```python
from build123d import *

# Parameters (mm, degrees)
SKETCH1_W                 = 25
SKETCH1_H                 = 10
CUT_EXTRUDE1_DEPTH        = 37.742346142
CUT_EXTRUDE1_DEPTH_BACK   = 37.742346142
SKETCH2_R                 = 105
F_3_0MM_DOWEL_HOLE1_D     = 3
F_3_0MM_DOWEL_HOLE1_DEPTH = 6


with BuildPart() as part:
    # Sketch1 → Revolve1 (revolve)
    with BuildSketch(Plane.XY, mode=Mode.PRIVATE) as revolve1_sk:
        with Locations((12.5, 5)):
            Rectangle(SKETCH1_W, SKETCH1_H)
    revolve(revolve1_sk.sketch.rotate(Axis((0, 0, 0), (0, 1, 0)), 90), axis=Axis((0, 0, 0), (0, 1, 0)))

    # Sketch2 → Cut-Extrude1 (cut, two sides: drawn at the far end of the back side and taken through both)
    with BuildSketch(Plane.XY.offset(-CUT_EXTRUDE1_DEPTH_BACK)):
        with Locations((0, 113)):
            Circle(SKETCH2_R)
    extrude(amount=CUT_EXTRUDE1_DEPTH + CUT_EXTRUDE1_DEPTH_BACK, mode=Mode.SUBTRACT)

    # Ø3.0mm Dowel Hole1
    with Locations(Plane(origin=(0, 0, 0), x_dir=(-1, 0, 0), z_dir=(0, -1, 0))):
        with Locations((17, 0)):
            Hole(F_3_0MM_DOWEL_HOLE1_D / 2, depth=F_3_0MM_DOWEL_HOLE1_DEPTH)


solid = part.part
```
The listing builds one solid part. Answer for the finished solid, in the listing's coordinates (mm). A direction names the side the tool comes from. Coordinates: 2 decimals unless noted, no trailing zeros. Loops run counter-clockwise (first coordinate to the right, second up) from the corner with the lowest first, then second, coordinate; pieces in that order, holes last. Notation, with made-up numbers: (-21, 19) -> (-16, 19) arc R21 ccw to (-16, 52) -> close; hole circle Ø5 at (18, 89.5). An arc over 180 degrees is marked (long way). Return JSON: item names as keys, results as strings. Group by question number.
(1) A cutting plane is placed at C-C on y = 6.75. Write down the section's boundary in (x, z).
(2) Given pin 1 Ø2 at (x, z) = (-16, -11) entering from +Y; pin 2 Ø2.5 at (x, z) = (-17, 0) entering from -Y; pin 3 Ø4 at (y, z) = (5, -7.5) entering from -X; pin 4 Ø4 at (x, z) = (19.5, -14) entering from +Y, each flat-ended and moving along its own axis, determine where each tip first touches the part or whether it passes through.
(3) Which of the six approach directions +Z, -Z, +X, -X, +Y, -Y give full straight-line access (tool end or side, diameter ignored) to faces 4 (the flat face through (-22, 10, 0)), 5 (the cylindrical face through (-18.5, 3.04, -0.07))?
(4) Determine the mould class of faces 1 (the cylindrical face through (9.58, 5.07, -23.09)), 2 (the flat face through (22, 10, 0)), 3 (the cylindrical face through (0, 8, 0)) for opening direction X: released by +X, released by -X, zero draft, split by the parting line, or undercut.
(5) A cutting plane is placed at B-B on y = 1.5. Write down the section's boundary in (x, z), and give its area (3 significant figures).
(6) A cutting plane is placed at A-A on z = 0. Write down the section's boundary in (x, y), and give its area (3 significant figures).
(7) Find the intervals of material crossed by probe 1 along Z at (x, y) = (-17, 4.65); probe 2 along X at (y, z) = (7, 15); probe 3 along Y at (x, z) = (-3, 23), in increasing order. Write a range as from..to.
(8) A cutting plane is placed at D-D on x = -17. Write down the section's boundary in (y, z), and give its area (3 significant figures).
The answers:
{
 "1": {"outline": "circle Ø50 at (0, 0)"},
 "2": {"pin 1": "stops at y = 9.39", "pin 2": "stops at y = 6", "pin 3": "stops at x = -24.39", "pin 4": "stops at y = 10"},
 "3": {"face 4": "+Z, -Z, +X, -X, +Y", "face 5": "-Y"},
 "4": {"face 1": "split by the parting line", "face 2": "zero draft", "face 3": "undercut"},
 "5": {"outline": "circle Ø50 at (0, 0); hole circle Ø3 at (-17, 0)", "area": "1,960 mm^2"},
 "6": {"outline": "(-25, 0) -> (-18.5, 0) -> (-18.5, 6) -> (-15.5, 6) -> (-15.5, 0) -> (25, 0) -> (25, 10) -> (20.4, 10) arc R105 cw to (-20.4, 10) -> (-25, 10) -> close", "area": "428 mm^2"},
 "7": {"probe 1": "z = -18.33..-1.5, 1.5..18.33", "probe 2": "x = -20..20", "probe 3": "y = 0..8.04"},
 "8": {"outline": "(0, -18.33) -> (9.39, -18.33) -> (9.39, 18.33) -> (0, 18.33) -> (0, 1.5) -> (6, 1.5) -> (6, -1.5) -> (0, -1.5) -> close", "area": "326 mm^2"}
}
